from build123d import *

# Parameters (mm, degrees)
F1_DEPTH = 9.525
F2_R     = 7.9375
F3_DEPTH = 25.4
F4_R     = 2.032
F5_DEPTH = 34.926
F6_R     = 1.143
F7_DEPTH = 25.4


with BuildPart() as f1:
    # F0 (on Front) → F1 (new body)
    with BuildSketch(Plane.XZ):
        with BuildLine():
            Line((7.9375, -19.05), (7.9375, 19.05))
            Line((7.9375, 19.05), (2.159, 19.05))
            ThreePointArc((2.159, 19.05), (0, 16.891), (-2.159, 19.05))
            Line((-2.159, 19.05), (-7.9375, 19.05))
            Line((-7.9375, 19.05), (-7.9375, -19.05))
            Line((-7.9375, -19.05), (-2.159, -19.05))
            ThreePointArc((-2.159, -19.05), (0, -16.891), (2.159, -19.05))
            Line((2.159, -19.05), (7.9375, -19.05))
        make_face()
        with BuildLine():
            Line((2.159, 19.05), (7.9375, 19.05))
            ThreePointArc((7.9375, 19.05), (0, 26.9875), (-7.9375, 19.05))
            Line((-7.9375, 19.05), (-2.159, 19.05))
            ThreePointArc((-2.159, 19.05), (0, 21.209), (2.159, 19.05))
        make_face()
        with BuildLine():
            ThreePointArc((-7.9375, -19.05), (0, -26.9875), (7.9375, -19.05))
            Line((7.9375, -19.05), (2.159, -19.05))
            ThreePointArc((2.159, -19.05), (0, -21.209), (-2.159, -19.05))
            Line((-2.159, -19.05), (-7.9375, -19.05))
        make_face()
    extrude(amount=F1_DEPTH)

    # F2 (on face) → F3 (join)
    with BuildSketch(Plane.XZ.offset(9.525)):
        Circle(F2_R)
    extrude(amount=F3_DEPTH)

    # F4 (on face) → F5 (cut, through all)
    with BuildSketch(Plane.XZ.offset(34.925)):
        Circle(F4_R)
    extrude(amount=-F5_DEPTH, mode=Mode.SUBTRACT)

    # F6 (on face) → F7 (cut)
    with BuildSketch(Plane(origin=(-7.9375, 0, 0), x_dir=(0, -1, 0), z_dir=(-1, 0, 0))):
        with Locations((22.225, 0)):
            Circle(F6_R)
    extrude(amount=-F7_DEPTH, mode=Mode.SUBTRACT)


solid = f1.part
Check sheet for the modelled part. Datum: model origin and axes. Units: mm. A direction names the side the tool comes from. Give positions to 0.01 mm unless a question says otherwise; leave off trailing zeros. Write each loop counter-clockwise with the first axis right and the second up, starting at its lowest first coordinate (ties: lowest second). Pieces come first, ordered by that corner, then holes. Notation, with made-up numbers: (29.5, 4) -> (47.5, 4) arc R10 ccw to (47.5, 9) -> close; hole circle Ø10 at (27, 33.25). An arc over 180 degrees is marked (long way). One line per item, written item: value. Start each with the question number.
Item 1: Tool access check on faces 1 (the flat face through (2, -34.925, -2)), 2 (the cylindrical face through (7.571, -22.047, 2.384)). Record the directions out of +Z, -Z, +X, -X, +Y, -Y that give a thin tool (end or side, any length) a straight path to the whole face; none if there is none.
Item 2: Section check C-C on z = 17.5. Record the cut outline in (x, y) (1 decimal).
Item 3: Section check B-B on x = 0. Record the cut outline in (y, z) (1 decimal), then the cut area to 3 significant figures.
Item 4: Draft check along X on faces 3 (the flat face through (-7.938, -5, 0)), 4 (the cylindrical face through (1.16, -4.7, -20.87)), 5 (the flat face through (0, -9.525, -16)). Enter one of: +X half, -X half, draft (parallel to the pull), parting line (faces both ways), or undercut.
Item 5: Section check A-A on y = -7. State how many separate pieces and enclosed holes the cut face has, then the cut area to 3 significant figures.
Item 6: Gauge pin test, flat ends, axial feed: pin 1 (5 mm diameter, centred on x = -2.5, z = 10.5, fed in from -Y) (3 decimals); pin 2 (6 mm diameter, centred on x = 3.5, y = -24, fed in from -Z); pin 3 (1.5 mm diameter, centred on x = -5, y = -17, fed in from +Z); pin 4 (2.5 mm diameter, centred on y = -22.225, z = 0, fed in from +X). Record the tip position at first contact, or that the pin passes through.
Item 7: Material ranges on probe 1 along Z at (x, y) = (0, -6.5); probe 2 along Y at (x, z) = (4.5, 0) (3 decimals); probe 3 along Y at (x, z) = (-0.5, 10.5) (3 decimals), recorded low to high. Write a range as from..to.
Item 8: Section check D-D on x = 5.5. Record the cut outline in (y, z) (3 decimals).
Results list:
1. face 1: +Z, -Z, +X, -X, -Y
1. face 2: -Y
2. outline: (-7.9, -9.5) -> (-1.5, -9.5) -> (-1.5, 0) -> (-7.9, 0) -> close; (1.5, -9.5) -> (7.9, -9.5) -> (7.9, 0) -> (1.5, 0) -> close
3. outline: (-34.9, -7.9) -> (-9.5, -7.9) -> (-9.5, -16.9) -> (0, -16.9) -> (0, -2) -> (-34.9, -2) -> close; (-34.9, 2) -> (0, 2) -> (0, 16.9) -> (-9.5, 16.9) -> (-9.5, 7.9) -> (-34.9, 7.9) -> close; (-9.5, -27) -> (0, -27) -> (0, -21.2) -> (-9.5, -21.2) -> close; (-9.5, 21.2) -> (0, 21.2) -> (0, 27) -> (-9.5, 27) -> close
3. area: 693 mm²
4. face 3: -X half
4. face 4: undercut
4. face 5: draft
5. separate pieces: 1
5. enclosed holes: 3
5. area: 761 mm²
6. pin 1: y = -9.525
6. pin 2: z = -7.92
6. pin 3: z = 6.7
6. pin 4: x = 7.94
7. probe 1: -26.99..-21.21, -16.89..-2.03, 2.03..16.89, 21.21..26.99
7. probe 2: -34.925..-23.368, -21.082..0
7. probe 3: -9.525..0
8. outline: (-34.925, -5.723) -> (-9.525, -5.723) -> (-9.525, -24.773) -> (0, -24.773) -> (0, 24.773) -> (-9.525, 24.773) -> (-9.525, 5.723) -> (-34.925, 5.723) -> close; hole circle Ø2.286 at (-22.225, 0)
